```python
from build123d import *


with BuildPart() as part:
    # body_sketch → body (revolve)
    with BuildSketch(Plane(origin=(0, 0, 0), x_dir=(1, 0, 0), z_dir=(0, 1, 0)), mode=Mode.PRIVATE) as body_sk:
        Polygon((0, 0), (12.1, 0), (12.5, -0.4), (12.5, -11.5), (12, -12), (10.5, -12), (2, -22.13), (0, -22.13), align=None)
    revolve(body_sk.sketch.rotate(Axis((0, 0, 0), (0, 0, 1)), 180), axis=Axis((0, 0, 0), (0, 0, 1)))

    # socket_sketch → socket (revolve, cut)
    with BuildSketch(Plane(origin=(0, 0, 0), x_dir=(1, 0, 0), z_dir=(0, 1, 0)), mode=Mode.PRIVATE) as socket_sk:
        Polygon((0, 0.5), (11.419545903, 0.5), (2.080454097, -10.63), (0, -10.63), align=None)
    revolve(socket_sk.sketch.rotate(Axis((0, 0, 0), (0, 0, 1)), 180), axis=Axis((0, 0, 0), (0, 0, 1)), mode=Mode.SUBTRACT)


solid = part.part
```
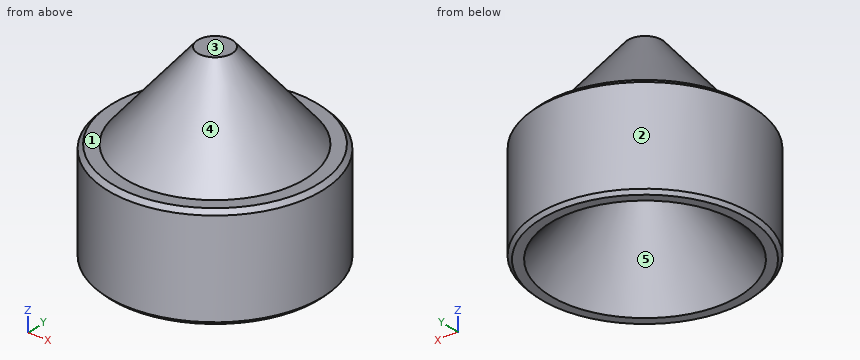
Work out the finished part from the listing and answer in its coordinate system (mm). Face numbers are marked on the shaded views. A direction names the side the tool comes from. Coordinates: 2 decimals unless noted, no trailing zeros. Write each loop counter-clockwise with the first axis right and the second up, starting at its lowest first coordinate (ties: lowest second). Pieces come first, ordered by that corner, then holes.
Q1. A cutting plane is placed at D-D, the plane z = 12.75. Give the vertices of the cut face in (x, y), then the cut area to 3 significant figures.
Q2. A cutting plane is placed at C-C, the plane z = 20.75. Give the vertices of the cut face in (x, y), then the cut area to 3 significant figures.
Q3. Find the intervals of material crossed by line 1 (Y direction, x = -1, z = 6.75); line 2 (X direction, y = 1.75, z = 6); line 3 (X direction, y = -6.75, z = 2.75), in increasing order.
Q4. Which of the six approach directions +Z, -Z, +X, -X, +Y, -Y give full straight-line access (tool end or side, diameter ignored) to the marked faces 1 and 2?
Q5. Determine the mould class of the marked faces 3, 4 and 5 for opening direction X: released by +X, released by -X, zero draft, split by the parting line, or undercut.
Q6. A cutting plane is placed at A-A, the plane x = 0. Give the vertices of the cut face in (y, z), then the cut area to 3 significant figures.
Q7. Each of these flat-tipped pins is pushed along its axis until it touches: pin 1 Ø3.5 at (x, y) = (-0.5, -1) entering from -Z; pin 2 Ø12 at (x, z) = (-8, 11) entering from +Y; pin 3 Ø1.5 at (x, y) = (7.5, -10) entering from +Z. Where does it stop, or does it pass through?
Findings below:
1. outline: circle Ø19.74 at (0, 0)
1. area: 306 mm2
2. outline: circle Ø6.32 at (0, 0)
2. area: 31.3 mm2
3. line 1: y = -12.46 to -5.24, 5.24 to 12.46
3. line 2: x = -12.38 to -5.7, 5.7 to 12.38
3. line 3: x = -10.52 to -5.48, 5.48 to 10.52
4. face 1: +Z
4. face 2: +Z, -Z
5. face 3: zero draft
5. face 4: split by the parting line
5. face 5: undercut
6. outline: (-12.5, 0.4) - (-12.1, 0) - (-11, 0) - (-2.08, 10.63) - (2.08, 10.63) - (11, 0) - (12.1, 0) - (12.5, 0.4) - (12.5, 11.5) - (12, 12) - (10.5, 12) - (2, 22.13) - (-2, 22.13) - (-10.5, 12) - (-12, 12) - (-12.5, 11.5) - close
6. area: 287 mm2
7. pin 1: stops at z = 9.69
7. pin 2: stops at y = 12.34
7. pin 3: stops at z = 12
